```python
from build123d import *


with BuildPart() as part:
    # Sketch1 → Revolve1 (revolve)
    with BuildSketch(Plane(origin=(0, 0, 0), x_dir=(1, 0, 0), z_dir=(0, 1, 0)), mode=Mode.PRIVATE) as revolve1_sk:
        with BuildLine():
            Line((-47.5, 1.5), (-47.5, 0.8))
            ThreePointArc((-47.5, 0.8), (-47.412132034, 0.587867966), (-47.2, 0.5))
            Line((-47.2, 0.5), (-46.5, 0.5))
            Line((-46.5, 0.5), (-22.5, 0.5))
            Line((-22.5, 0.5), (-21.8, 0.5))
            ThreePointArc((-21.8, 0.5), (-21.587867966, 0.587867966), (-21.5, 0.8))
            Line((-21.5, 0.8), (-21.5, 1.5))
            Line((-21.5, 1.5), (-21.5, 4))
            Line((-21.5, 4), (-21.2, 4))
            Line((-21.2, 4), (-21.2, 0.8))
            ThreePointArc((-21.2, 0.8), (-21.375735931, 0.375735931), (-21.8, 0.2))
            Line((-21.8, 0.2), (-47.2, 0.2))
            ThreePointArc((-47.2, 0.2), (-47.624264069, 0.375735931), (-47.8, 0.8))
            Line((-47.8, 0.8), (-47.8, 4))
            Line((-47.8, 4), (-47.5, 4))
            Line((-47.5, 4), (-47.5, 1.5))
        make_face()
    revolve(revolve1_sk.sketch.rotate(Axis((0, 0, 0), (0, 0, -1)), 180), axis=Axis((0, 0, 0), (0, 0, -1)))


solid = part.part
```
Check sheet for the modelled part. Datum: model origin and axes. Units: mm. Round coordinates to 2 decimals unless told otherwise and drop trailing zeros. Order: outer loops, then holes, each group sorted by start corner. A loop starts at its lowest first (then second) coordinate and runs counter-clockwise, first axis right, second up. Notation, with made-up numbers: (87.5, 4) -> (125.5, 4) arc R18 ccw to (125.5, 24) -> close; hole circle Ø8 at (53, -20). An arc over 180 degrees is marked (long way). One line per item, written item: value. Start each with the question number.
Q1. Mould release check, pull along Y, two halves, no side actions. Record for faces 1 (the face through (-16.824, 12.9, -2.378)), 2 (the face through (-2.799, -21.317, -2.422)), 3 (the face through (25.697, -40.305, -2.422)), 4 (the face through (-20, 10, -0.2)): pulls with the +Y half, pulls with the -Y half, needs draft (parallel to the pull), parting line crosses it, or undercut.
Q2. Gauge pin test, flat ends, axial feed: pin 1 Ø1 at (x, z) = (33, -3.5) entering from +Y; pin 2 Ø6 at (x, y) = (-26, 18) entering from -Z; pin 3 Ø8 at (x, y) = (-33, 36.5) entering from -Z; pin 4 Ø1.5 at (y, z) = (29.5, -2) entering from -X. Record the tip position at first contact, or that the pin passes through.
Q3. Cross-section at C-C (z = -2.5). Record the boundary of the cut face in (x, y).
Q4. Thickness scan on line 1 (Y direction, x = 0, z = -1.55); line 2 (Y direction, x = 5.5, z = -0.75); line 3 (X direction, y = -12, z = -3.7). Record the ranges inside material, lowest first.
Q5. Cross-section at A-A (x = 0). Record the boundary of the cut face in (y, z), and give its area (3 significant figures).
Completed:
1. face 1: undercut
1. face 2: undercut
1. face 3: parting line crosses it
1. face 4: needs draft
2. pin 1: stops at y = 35.05
2. pin 2: stops at z = -0.5
2. pin 3: stops at z = -4
2. pin 4: stops at x = -38.19
3. outline: circle Ø95.6 at (0, 0); circle Ø43 at (0, 0); hole circle Ø95 at (0, 0); hole circle Ø42.4 at (0, 0)
4. line 1: y = -47.8 to -47.5, -21.5 to -21.2, 21.2 to 21.5, 47.5 to 47.8
4. line 2: y = -47.48 to -47.18, -20.79 to -20.48, 20.48 to 20.79, 47.18 to 47.48
4. line 3: x = -46.27 to -45.96, -17.84 to -17.48, 17.48 to 17.84, 45.96 to 46.27
5. outline: (-47.8, -4) -> (-47.5, -4) -> (-47.5, -0.8) arc R0.3 cw to (-47.2, -0.5) -> (-21.8, -0.5) arc R0.3 cw to (-21.5, -0.8) -> (-21.5, -4) -> (-21.2, -4) -> (-21.2, -0.8) arc R0.6 ccw to (-21.8, -0.2) -> (-47.2, -0.2) arc R0.6 ccw to (-47.8, -0.8) -> close; (21.2, -4) -> (21.5, -4) -> (21.5, -0.8) arc R0.3 cw to (21.8, -0.5) -> (47.2, -0.5) arc R0.3 cw to (47.5, -0.8) -> (47.5, -4) -> (47.8, -4) -> (47.8, -0.8) arc R0.6 ccw to (47.2, -0.2) -> (21.8, -0.2) arc R0.6 ccw to (21.2, -0.8) -> close
5. area: 19.9 mm²
